from build123d import *

# Parameters (mm, degrees)
F1_DEPTH  = 2133.6
F2_DEPTH  = 2133.6
F3_DEPTH  = 2133.6
F4_DEPTH  = 1905
F5_W      = 673.1
F5_H      = 419.1
F5_H_2    = 1574.8
F6_DEPTH  = 19.05
F7_DEPTH  = 209.55
F8_DEPTH  = 1663.7
F9_DEPTH  = 1644.65
F10_DEPTH = 1231.9
F11_DEPTH = 1212.85
F12_DEPTH = 787.4
F13_DEPTH = 768.35
F14_DEPTH = 393.7
F15_DEPTH = 374.65
F16_DEPTH = 50.8
F17_DEPTH = 31.75
F18_DEPTH = 50.8
F19_DEPTH = 50.8
F20_DEPTH = 50.8
F21_DEPTH = 50.8
F22_DEPTH = 12.7


with BuildPart() as f1:
    # F0 (on Top) → F1 (new body)
    with BuildSketch(Plane.XY):
        Polygon((-354.0592090795, -381), (-380.9999747663, -381), (-380.9999747663, -400.05), (381.0000252337, -400.05), (381.0000252337, -381), (354.0592559783, -381), align=None)
    extrude(amount=F1_DEPTH)

    # F0 (on Top) → F2 (join)
    with BuildSketch(Plane.XY):
        Polygon((381.0000252337, -381), (0, 0), (0, -26.9407674711), (354.0592559783, -381), align=None)
        Polygon((0, 0), (-380.9999747663, -381), (-354.0592090795, -381), (0, -26.9407674711), align=None)
    extrude(amount=F2_DEPTH)

    # F0 (on Top) → F3 (join)
    with BuildSketch(Plane.XY):
        Polygon((0, -26.9407674711), (-354.0592090795, -381), (354.0592559783, -381), align=None)
    extrude(amount=F3_DEPTH)

    # F0 (on Top) → F4 (cut)
    with BuildSketch(Plane.XY):
        Polygon((0, -26.9407674711), (-354.0592090795, -381), (354.0592559783, -381), align=None)
    extrude(amount=F4_DEPTH, mode=Mode.SUBTRACT)

    # F5 (on face) → F6 (cut)
    with BuildSketch(Plane.XZ.offset(400.05)):
        with Locations((2.52337e-05, 1873.25)):
            Rectangle(F5_W, F5_H)
        with Locations((2.52337e-05, 838.2)):
            Rectangle(F5_W, F5_H_2)
    extrude(amount=-F6_DEPTH, mode=Mode.SUBTRACT)

    # F7 (cut): a face of the model
    f7_faces = [f1.faces().sort_by_distance(p)[0] for p in [
        (1.56329e-05, -262.9802558237, 1905),
    ]]
    extrude(f7_faces, amount=-F7_DEPTH, mode=Mode.SUBTRACT)

    # F0 (on Top) → F8 (join)
    with BuildSketch(Plane.XY):
        Polygon((0, -26.9407674711), (-354.0592090795, -381), (354.0592559783, -381), align=None)
    extrude(amount=F8_DEPTH)

    # F0 (on Top) → F9 (cut)
    with BuildSketch(Plane.XY):
        Polygon((0, -26.9407674711), (-354.0592090795, -381), (354.0592559783, -381), align=None)
    extrude(amount=F9_DEPTH, mode=Mode.SUBTRACT)

    # F0 (on Top) → F10 (join)
    with BuildSketch(Plane.XY):
        Polygon((0, -26.9407674711), (-354.0592090795, -381), (354.0592559783, -381), align=None)
    extrude(amount=F10_DEPTH)

    # F0 (on Top) → F11 (cut)
    with BuildSketch(Plane.XY):
        Polygon((0, -26.9407674711), (-354.0592090795, -381), (354.0592559783, -381), align=None)
    extrude(amount=F11_DEPTH, mode=Mode.SUBTRACT)

    # F0 (on Top) → F12 (join)
    with BuildSketch(Plane.XY):
        Polygon((0, -26.9407674711), (-354.0592090795, -381), (354.0592559783, -381), align=None)
    extrude(amount=F12_DEPTH)

    # F0 (on Top) → F13 (cut)
    with BuildSketch(Plane.XY):
        Polygon((0, -26.9407674711), (-354.0592090795, -381), (354.0592559783, -381), align=None)
    extrude(amount=F13_DEPTH, mode=Mode.SUBTRACT)

    # F0 (on Top) → F14 (join)
    with BuildSketch(Plane.XY):
        Polygon((0, -26.9407674711), (-354.0592090795, -381), (354.0592559783, -381), align=None)
    extrude(amount=F14_DEPTH)

    # F0 (on Top) → F15 (cut)
    with BuildSketch(Plane.XY):
        Polygon((0, -26.9407674711), (-354.0592090795, -381), (354.0592559783, -381), align=None)
    extrude(amount=F15_DEPTH, mode=Mode.SUBTRACT)

    # F0 (on Top) → F16 (join)
    with BuildSketch(Plane.XY):
        Polygon((0, -26.9407674711), (-354.0592090795, -381), (354.0592559783, -381), align=None)
    extrude(amount=F16_DEPTH)

    # F0 (on Top) → F17 (cut)
    with BuildSketch(Plane.XY):
        Polygon((0, -26.9407674711), (-354.0592090795, -381), (354.0592559783, -381), align=None)
    extrude(amount=F17_DEPTH, mode=Mode.SUBTRACT)

    # F18 (add): a face of the model
    f18_faces = [f1.faces().sort_by_distance(p)[0] for p in [
        (1.56329e-05, -262.9802558237, 787.4),
    ]]
    extrude(f18_faces, amount=F18_DEPTH)

    # F19 (cut): a face of the model
    f19_faces = [f1.faces().sort_by_distance(p)[0] for p in [
        (1.56329e-05, -262.9802558237, 768.35),
    ]]
    extrude(f19_faces, amount=-F19_DEPTH, mode=Mode.SUBTRACT)

    # F20 (add): a face of the model
    f20_faces = [f1.faces().sort_by_distance(p)[0] for p in [
        (1.56329e-05, -262.9802558237, 393.7),
    ]]
    extrude(f20_faces, amount=F20_DEPTH)

    # F21 (cut): a face of the model
    f21_faces = [f1.faces().sort_by_distance(p)[0] for p in [
        (1.56329e-05, -262.9802558237, 374.65),
    ]]
    extrude(f21_faces, amount=-F21_DEPTH, mode=Mode.SUBTRACT)

    # F0 (on Top) → F22 (cut)
    with BuildSketch(Plane.XY):
        Polygon((381.0000252337, -381), (0, 0), (0, -26.9407674711), (354.0592559783, -381), align=None)
        Polygon((0, 0), (-380.9999747663, -381), (-354.0592090795, -381), (0, -26.9407674711), align=None)
        Polygon((-354.0592090795, -381), (-380.9999747663, -381), (-380.9999747663, -400.05), (381.0000252337, -400.05), (381.0000252337, -381), (354.0592559783, -381), align=None)
    extrude(amount=F22_DEPTH, mode=Mode.SUBTRACT)


solid = f1.part
Design review of the part built by this model. Coordinates are the model's own, in mm. A direction names the side the tool comes from. Give positions to 0.01 mm unless a question says otherwise; leave off trailing zeros. Write each loop counter-clockwise with the first axis right and the second up, starting at its lowest first coordinate (ties: lowest second). Pieces come first, ordered by that corner, then holes. Notation, with made-up numbers: M -15,10.25 L 11,10.25 A26 cw 11,29.25 Z; hole C 33,87 d9. An arc over 180 degrees is marked long. Return JSON: item names as keys, results as strings. Group by question number.
Item 1: Tool access review of faces 5 (the flat face through (-2, -381, 2088)), 6 (the flat face through (193, -193, 1058)), 7 (the flat face through (179.51, -206.45, 22.09)): name each direction out of +Z, -Z, +X, -X, +Y, -Y from which nothing blocks a thin tool from reaching the whole face with its end or side.
Item 2: The part is to be moulded in two halves that separate along Y. For faces 1 (the flat face through (-188, -188, 1058)), 2 (the flat face through (-340, -400.05, 990)), 3 (the flat face through (-174.55, -201.49, 22.09)), 4 (the flat face through (-5, -241, 2114.55)), say which applies: pulls with the +Y half, pulls with the -Y half, needs draft (parallel to the pull), parting line crosses it, or undercut.
Item 3: Clearance check with flat-ended pins moving along their axes: pin 1 Ø12 at (x, z) = (57, 421.5) entering from +Y; pin 2 Ø5.5 at (x, z) = (346.5, 1030.5) entering from +Y; pin 3 Ø14 at (x, z) = (-342, 714.5) entering from +Y. State where each tip first meets the part, or that it passes through.
Item 4: Take a section at A-A (y = -250). Give the boundary of the cut face in (x, z), plus the area to 3 significant figures.
Item 5: Take a section at D-D (y = -128). Give the boundary of the cut face in (x, z), plus the area to 3 significant figures.
Item 6: Wall thickness on line 1 along Z through (x, y) = (65, -310.5); line 2 along Z through (x, y) = (88.5, -381.5); line 3 along X through (y, z) = (-248.5, 2001.5): over which ranges is each line inside the solid? List them lowest first.
Item 7: Take a section at B-B (z = 1530). Give the boundary of the cut face in (x, y).
Return value:
{
 "1": {"face 5": "none", "face 6": "+Z, -Z, +X, +Y", "face 7": "-Z"},
 "2": {"face 1": "pulls with the +Y half", "face 2": "pulls with the -Y half", "face 3": "undercut", "face 4": "undercut"},
 "3": {"pin 1": "stops at y = -51", "pin 2": "stops at y = -343.75", "pin 3": "stops at y = -335"},
 "4": {"outline": "M -250,12.7 L -223.06,12.7 L -223.06,31.75 L 223.06,31.75 L 223.06,12.7 L 250,12.7 L 250,2133.6 L -250,2133.6 Z; hole M -223.06,50.8 L 223.06,50.8 L 223.06,425.45 L -223.06,425.45 Z; hole M -223.06,444.5 L 223.06,444.5 L 223.06,819.15 L -223.06,819.15 Z; hole M -223.06,838.2 L 223.06,838.2 L 223.06,1212.85 L -223.06,1212.85 Z; hole M -223.06,1231.9 L 223.06,1231.9 L 223.06,1644.65 L -223.06,1644.65 Z; hole M -223.06,1663.7 L 223.06,1663.7 L 223.06,2114.55 L -223.06,2114.55 Z", "area": "165,000 mm2"},
 "5": {"outline": "M -128,12.7 L -101.06,12.7 L -101.06,31.75 L 101.06,31.75 L 101.06,12.7 L 128,12.7 L 128,2133.6 L -128,2133.6 Z; hole M -101.06,50.8 L 101.06,50.8 L 101.06,425.45 L -101.06,425.45 Z; hole M -101.06,444.5 L 101.06,444.5 L 101.06,819.15 L -101.06,819.15 Z; hole M -101.06,838.2 L 101.06,838.2 L 101.06,1212.85 L -101.06,1212.85 Z; hole M -101.06,1231.9 L 101.06,1231.9 L 101.06,1644.65 L -101.06,1644.65 Z; hole M -101.06,1663.7 L 101.06,1663.7 L 101.06,2114.55 L -101.06,2114.55 Z", "area": "137,000 mm2"},
 "6": {"line 1": "z = 31.75 to 50.8, 425.45 to 444.5, 819.15 to 838.2, 1212.85 to 1231.9, 1644.65 to 1663.7, 2114.55 to 2133.6", "line 2": "z = 12.7 to 50.8, 1625.6 to 1663.7, 2082.8 to 2133.6", "line 3": "x = -248.5 to -221.56, 221.56 to 248.5"},
 "7": {"outline": "M -381,-400.05 L -336.55,-400.05 L -336.55,-381 L -354.06,-381 L 0,-26.94 L 354.06,-381 L 336.55,-381 L 336.55,-400.05 L 381,-400.05 L 381,-381 L 0,0 L -381,-381 Z"}
}
